```python
from build123d import *

# Parameters (mm, degrees)
F0_R     = 30
F0_R_2   = 13
F1_DEPTH = 15
F2_R     = 5
F3_SIZE  = 3
F4_SIZE  = 2


with BuildPart() as f1:
    # F0 (on Front) → F1 (new body)
    with BuildSketch(Plane.XZ):
        Circle(F0_R)
        Circle(F0_R_2, mode=Mode.SUBTRACT)
    extrude(amount=F1_DEPTH)

    # F2
    f2_edges = [f1.edges().sort_by_distance(p)[0] for p in [
        (-30, -15, 0),
    ]]
    fillet(f2_edges, radius=F2_R)

    # F3
    f3_edges = [f1.edges().sort_by_distance(p)[0] for p in [
        (-13, -15, 0),
    ]]
    chamfer(f3_edges, length=F3_SIZE)

    # F4
    f4_edges = [f1.edges().sort_by_distance(p)[0] for p in [
        (-30, 0, 0),
    ]]
    chamfer(f4_edges, length=F4_SIZE)


solid = f1.part
```
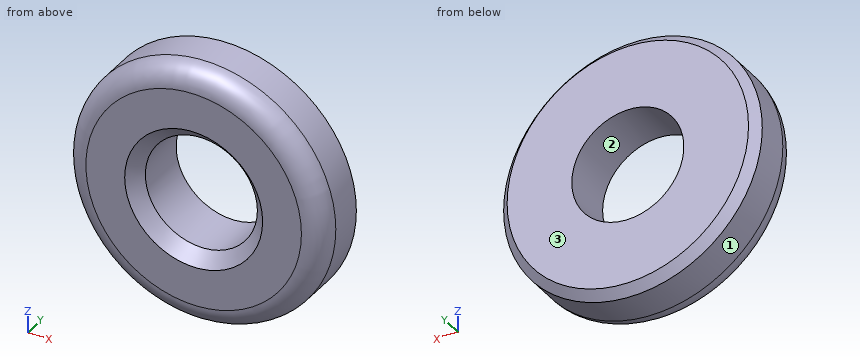
Check sheet for the modelled part. Datum: model origin and axes. Units: mm. Face numbers are marked on the shaded views. Coordinates: 2 decimals unless noted, no trailing zeros. Order: outer loops, then holes, each group sorted by start corner. A loop starts at its lowest first (then second) coordinate and runs counter-clockwise, first axis right, second up. Notation, with made-up numbers: (42, 30.5) -> (65, 30.5) arc R6 ccw to (65, 41.5) -> close; hole circle Ø6 at (-11, -23). An arc over 180 degrees is marked (long way). Write each question's results on one line, items separated by ' | '. Start each with the question number.
1) Material ranges on line 1 along Z through (x, y) = (0, -5.5); line 2 along X through (y, z) = (-12.25, 8); line 3 along Z through (x, y) = (1.5, -12.25), recorded low to high.
2) Section check C-C (y = -8.5). Enter the section's corners in (x, z).
3) Section check A-A (z = 0). Enter the section's corners in (x, y).
4) Depth check by flat-ended pin: pin 1 (6 mm diameter, centred on x = -12, y = -8, fed in from -Z); pin 2 (1 mm diameter, centred on x = 2.5, y = -6.5, fed in from -Z); pin 3 (6 mm diameter, centred on x = -13.5, z = 4.5, fed in from +Y); pin 4 (2 mm diameter, centred on y = -12.5, z = -5, fed in from +X). Enter the tip coordinate at first touch or a pass-through.
5) Section check B-B (x = 0). Enter the section's corners in (y, z).
6) Draft check along Z on the marked faces 1, 2 and 3. Enter one of: pulls with the +Z half, pulls with the -Z half, needs draft (parallel to the pull), parting line crosses it, or undercut.
Checked values:
1) line 1: -30 to -13, 13 to 30 | line 2: -28.36 to -10.56, 10.56 to 28.36 | line 3: -29.43 to -13.16, 13.16 to 29.43
2) outline: circle Ø60 at (0, 0); hole circle Ø26 at (0, 0)
3) outline: (-30, -10) arc R5 ccw to (-25, -15) -> (-16, -15) -> (-13, -12) -> (-13, 0) -> (-28, 0) -> (-30, -2) -> close; (13, -12) -> (16, -15) -> (25, -15) arc R5 ccw to (30, -10) -> (30, -2) -> (28, 0) -> (13, 0) -> close
4) pin 1: z = -28.62 | pin 2: z = -29.93 | pin 3: y = 0 | pin 4: x = 29.38
5) outline: (-15, -25) arc R5 ccw to (-10, -30) -> (-2, -30) -> (0, -28) -> (0, -13) -> (-12, -13) -> (-15, -16) -> close; (-15, 16) -> (-12, 13) -> (0, 13) -> (0, 28) -> (-2, 30) -> (-10, 30) arc R5 ccw to (-15, 25) -> close
6) face 1: parting line crosses it | face 2: undercut | face 3: needs draft
